Autodesk Inventor part; units mm, degrees
ref_plane "Plano de trabajo4" through (-5.75, -5, -2.5) normal (1, 0, 0) x (0, 0, -1)
ref_plane "YZ Plane" through (0, 0, 0) normal (1, 0, 0) x (0, 1, 0)
ref_plane "XZ Plane" through (0, 0, 0) normal (0, 1, 0) x (-1, 0, 0)
sketch "Boceto1" plane through (0, 0, 0) normal (0, 0, 1) x (1, 0, 0)
  line L0 (81, 20) -> (81, 63.5)
  line L1 (-27.5, 63.5) -> (-27.5, -5)
  line L2 (-27.5, -5) -> (16, -5)
  line L3 (16, -5) -> (16, 20)
  line L4 (11, 25) -> (11, -5)
  line L5 (-22.5, 58.5) -> (-22.5, -5)
  line L6 (11, 25) -> (81, 25)
  line L7 (-27.5, 63.5) -> (81, 63.5)
  line L8 (-22.5, 58.5) -> (81, 58.5)
  line L9 (16, 20) -> (81, 20)
  point P0 (0, 0)
  dimension "d7" = 5
  dimension "d68" = 5
  dimension "d69" = 33.5
  dimension "d74" = 5
  dimension "d75" = 33.5
  dimension "d76" = 5
  dimension "d77" = 70
  dimension "d111" = 30
extrude "Extrusión1" add sketch "Boceto1" against normal blind 2.5
extrude "Extrusión2" add sketch "Boceto1" along normal blind 1 contours L9 L3 L2 L4 L6 L0 | L8 L5 L2 L1 L7 L0
ref_plane "Plano de trabajo3" through (29.25, 58.5, 1) normal (0, 0, 1) x (1, 0, 0)
mirror "Simetría3" about plane through (29.25, 58.5, 1) normal (0, 0, 1) of "Extrusión2", "Extrusión1"
sketch "Boceto6" plane through (-27.5, 63.5, 4.5) normal (0, 0, 1) x (1, 0, 0)
  line L0 (108.5, -43.5) -> (43.5, -43.5)
  line L1 (0, -68.5) -> (0, 0)
  line L2 (0, -43.5) -> (0, -51.5)
  line L3 (43.5, -43.5) -> (43.5, -68.5)
  line L4 (0, -43.5) -> (38.5, -43.5)
  line L5 (38.5, -68.5) -> (38.5, -38.5)
  line L6 (0, -51.5) -> (38.5, -51.5)
  line L7 (38.5, -43.5) -> (38.5, -51.5)
  point P0 (27.5, -63.5)
  point P1 (43.5, -51.5)
  dimension "d78" = 8
extrude "Extrusión11" cut sketch "Boceto6" against normal blind 4.5
sketch "Boceto7" plane through (-27.5, -5, -2.5) normal (-1, 0, 0) x (0, 0, 1)
  line L0 (0, 0) -> (0, 68.5)
  line L1 (0, 0) -> (0, -42.4)
  line L2 (0, 0) -> (7, 0)
  line L3 (0, 0) -> (7, 0)
  line L4 (7, 0) -> (7, -42.4)
  line L5 (0, -42.4) -> (86.5, -192.2224)
  line L6 (86.5, -192.2224) -> (89, -192.2224)
  line L7 (89, -192.2224) -> (92.375, -190.2738)
  line L8 (2.5, 0) -> (2.5, -42.4)
  line L9 (0, 0) -> (7, 0)
  line L10 (0, 0) -> (2.5, 0)
  line L11 (86.5, -192.2224) -> (89, -192.2224)
  line L12 (89, -192.2224) -> (92.375, -190.2738)
  line L13 (2.5, -42.4) -> (89, -192.2224)
  line L14 (0, -42.4) -> (-1.0904, -42.4)
  line L15 (7, -42.4) -> (92.375, -190.2738)
  line L16 (86.5, -187.8923) -> (89.875, -185.9437)
  point P0 (2.5, 5)
  point P1 (4.5, 0)
  point P2 (-0.5452, -42.4)
  dimension "d81" = 42.4
  dimension "d82" = 173
  dimension "d88" = 120
  dimension "d108" = 5
ref_plane "Plano de trabajo4" through (-5.75, -5, -2.5) normal (1, 0, 0) x (0, 0, -1)
extrude "Extrusión12" add sketch "Boceto7" against normal blind 21.75 contours L2 L8 L13 L6 L5 L1
extrude "Extrusión13" add sketch "Boceto7" against normal blind 5 contours L2 L4 L15 L16 L13 L8
extrude "Extrusión14" add sketch "Boceto7" against normal blind 21.75 contours L13 L16 L15 L7
mirror "Simetría4" about plane through (-5.75, -5, -2.5) normal (1, 0, 0) of "Extrusión12", "Extrusión13", "Extrusión14"
sketch "Boceto8" plane through (-22.5, -47.4, 0) normal (0, 0.5, 0.866) x (1, 0, 0)
  line L0 (0, 0) -> (33.5, 0)
  line L1 (16.75, 0) -> (16.75, -5)
  circle A0 centre (16.75, -15.25) radius 10.25
  line L2 (16.75, -25.5) -> (16.75, -30.5)
  circle A1 centre (16.75, -41.5) radius 11
  line L3 (16.75, -52.5) -> (16.75, -57.5)
  circle A2 centre (16.75, -68.69) radius 11.19
  line L4 (16.75, -79.88) -> (16.75, -84.88)
  circle A3 centre (16.75, -96.38) radius 11.5
  line L5 (16.75, -107.88) -> (16.75, -112.88)
  circle A4 centre (16.75, -125.07) radius 12.19
  line L6 (16.75, -137.26) -> (16.75, -142.26)
  circle A5 centre (16.75, -155.01) radius 12.75
  point P0 (22.5, 41.0496)
  dimension "d105" = 25.5
  dimension "d94" = 5
  dimension "d95" = 20.5
  dimension "d96" = 5
  dimension "d97" = 5
  dimension "d98" = 5
  dimension "d99" = 5
  dimension "d100" = 5
  dimension "d101" = 22
  dimension "d102" = 22.38
  dimension "d103" = 23
  dimension "d104" = 24.38
extrude "Extrusión15" cut sketch "Boceto8" against normal blind 21.75
sketch "Boceto9" plane through (-27.5, 63.5, -2.5) normal (-1, 0, 0) x (0, 0, 1)
  line L0 (2.5, -51.5) -> (2.5, -110.9)
  line L1 (0, 0) -> (0, -110.9)
  line L2 (0, -110.9) -> (2.5, -110.9)
  line L3 (2.5, -110.9) -> (2.5, -70.9)
  line L4 (2.5, -70.9) -> (0, -70.9)
  line L5 (0, -70.9) -> (0, -110.9)
  line L6 (0, -43.5) -> (0, -110.9)
  line L7 (0, -102.4) -> (2.5, -102.4)
  point P0 (2.5, -63.5)
  point P1 (7, -110.9)
  dimension "d109" = 2.5
  dimension "d110" = 40
  dimension "d112" = 31.5
extrude "Extrusión16" cut sketch "Boceto9" against normal through all contours L0 L7 L1 L4
equation "\"d105\" = UnSol"
equation "\"d94\" = razon"
equation "\"d95\" = diezcen"
equation "\"d96\" = razon"
equation "\"d97\" = razon"
equation "\"d98\" = razon"
equation "\"d99\" = razon"
equation "\"d100\" = razon"
equation "\"d101\" = cincuentacen"
equation "\"d102\" = dossol"
equation "\"d103\" = veintecen"
equation "\"d104\" = cincosol"
equation "\"UnSol\" = 25.5"
equation "\"diezcen\" = 20.5"
equation "\"veintecen\" = 23"
equation "\"cincuentacen\" = 22"
equation "\"dossol\" = 22.38"
equation "\"cincosol\" = 24.38"
equation "\"razon\" = 5"
properties part number "Maquinita"
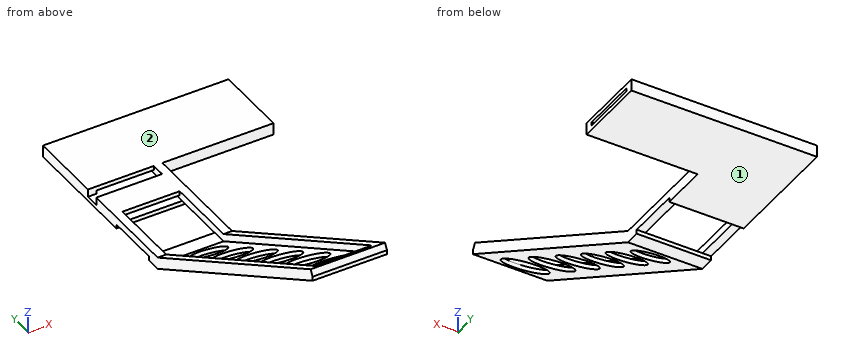
Geometry: final body of the model. Coordinates: model frame, mm. Face numbers are marked on the shaded views. A direction names the side the tool comes from. Give positions to 0.01 mm unless a question says otherwise; leave off trailing zeros. Order: outer loops, then holes, each group sorted by start corner. A loop starts at its lowest first (then second) coordinate and runs counter-clockwise, first axis right, second up. Notation, with made-up numbers: (63, 74.5) -> (80, 74.5) arc R16 ccw to (80, 99.5) -> close; hole circle Ø7 at (32, 22.5). An arc over 180 degrees is marked (long way). Answer as a JSON object with one key per item and string values.
Q1. Section B-B (y = 3). Output: boundary loops of the cut face in (x, z), plus the area to 4 significant figures.
Entries:
{"outline": "(-27.5, -2.5) -> (16, -2.5) -> (16, 4.5) -> (-27.5, 4.5) -> close; hole (-22.5, 0) -> (11, 0) -> (11, 2) -> (-22.5, 2) -> close", "area": "237.5 mm^2"}
Q2. First-contact query: pin 1 (2 mm diameter, centred on x = 0, z = 3.5, fed in from -Y); pin 2 (5.5 mm diameter, centred on x = 14.5, y = -18, fed in from -Z); pin 3 (9.5 mm diameter, centred on x = -1.5, y = -41.5, fed in from +Z); pin 4 (12 mm diameter, centred on y = 6.5, z = 8.5, fed in from -X). Flat tips, straight axial feed; report the tip coordinate or a pass-through.
Entries:
{"pin 1": "stops at y = -54.24", "pin 2": "stops at z = 0", "pin 3": "stops at z = 0", "pin 4": "stops at x = -27.5"}
Q3. Material intervals for probe 1 along X at (y, z) = (-115, 41.5); probe 2 along Z at (x, y) = (9, 6.5); probe 3 along Y at (x, z) = (5, 2.5), sorted ascending.
Entries:
{"probe 1": "x = -27.5 to -22.5, 11 to 16", "probe 2": "z = -2.5 to 0, 2 to 4.5", "probe 3": "y = -56.06 to -51.73, -5 to 12, 20 to 63.5"}
Q4. Section D-D (x = -9.5). State how many separate pieces and enclosed holes the cut face has, plus the area to 3 significant figures.
Entries:
{"separate pieces": "9", "enclosed holes": "0", "area": "472 mm^2"}
Q5. Access query for the marked faces 1 and 2. Directions: +Z, -Z, +X, -X, +Y, -Y. A direction counts if a zero-diameter tool reaches every point of the face in a straight line with its end or side. Return the directions, or none.
Entries:
{"face 1": "-Z, +X, -X, +Y, -Y", "face 2": "+Z, +X, -X, +Y"}
Q6. Section C-C (x = 65). Output: boundary loops of the cut face in (y, z).
Entries:
{"outline": "(20, -2.5) -> (63.5, -2.5) -> (63.5, 4.5) -> (20, 4.5) -> close; hole (25, 0) -> (58.5, 0) -> (58.5, 2) -> (25, 2) -> close"}
Q7. Section A-A (y = -29.5). Output: boundary loops of the cut face in (x, z), plus the area to 3 significant figures.
Entries:
{"outline": "(-27.5, 0) -> (-22.5, 0) -> (-22.5, 4.5) -> (-27.5, 4.5) -> close; (11, 0) -> (16, 0) -> (16, 4.5) -> (11, 4.5) -> close", "area": "45.0 mm^2"}
